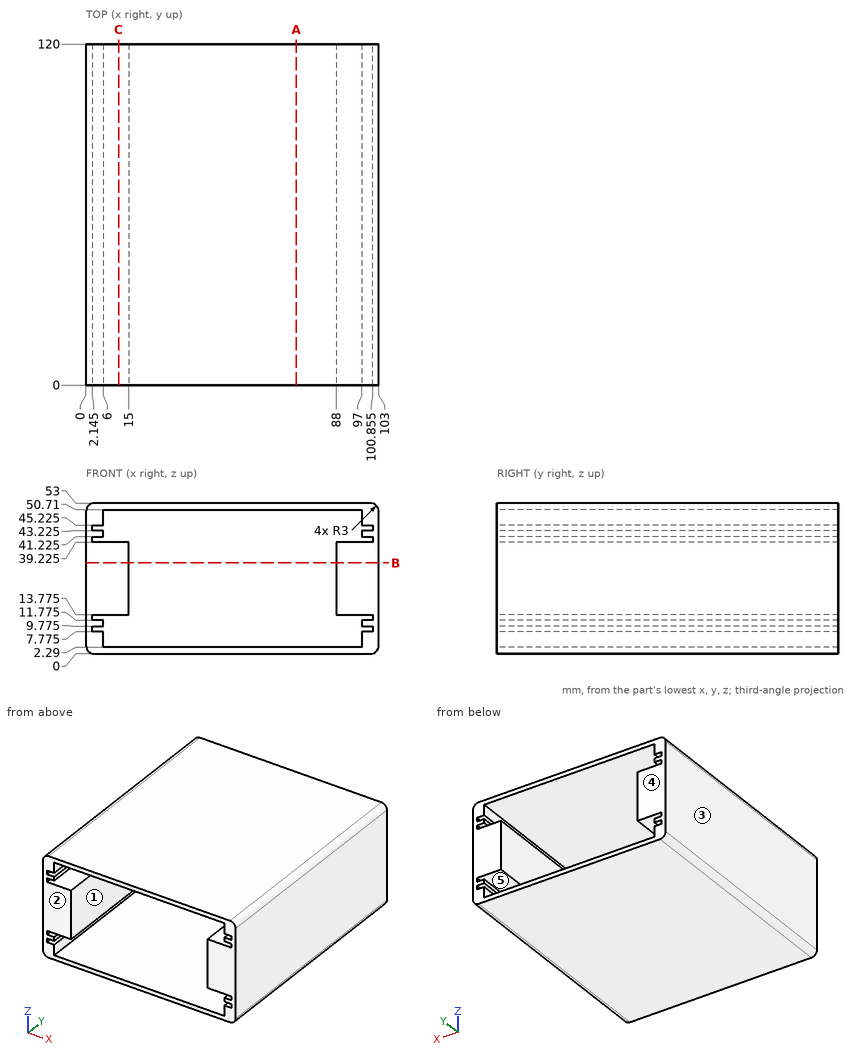
Geometry: see drawing. Coordinates: mm, zero at the bounding-box minimum. A direction names the side the tool comes from. Give positions to 0.01 mm unless a question says otherwise; leave off trailing zeros. Order: outer loops, then holes, each group sorted by start corner. A loop starts at its lowest first (then second) coordinate and runs counter-clockwise, first axis right, second up.
Q1. Draft query along X for the marked faces 1, 2 and 3. Return one class per face: +X half, -X half, draft (parallel to the pull), parting line (faces both ways), or undercut.
Checked values:
face 1: undercut
face 2: draft
face 3: -X half
Q2. Section B-B on z = 32. Output: boundary loops of the cut face in (x, y), and give its area (3 significant figures).
Checked values:
outline: (0, 0) - (15, 0) - (15, 120) - (0, 120) - close; (88, 0) - (103, 0) - (103, 120) - (88, 120) - close
area: 3,600 mm2
Q3. Set-up query: the marked faces 4 and 5. Return all of +Z, -Z, +X, -X, +Y, -Y with unobstructed straight access to the full face (end or side cutting, diameter ignored); none if empty.
Checked values:
face 4: +Z, -Z, +X, -X, +Y
face 5: +Y, -Y
Q4. Ray query, probe 1 along Z at (x, y) = (11, 114) (3 decimals); probe 2 along Z at (x, y) = (5, 32) (3 decimals); probe 3 along Z at (x, y) = (22.5, 94). Return the intervals inside material, ascending.
Checked values:
probe 1: z = 0 to 2.29, 13.775 to 39.225, 50.71 to 53
probe 2: z = 0 to 7.775, 9.775 to 11.775, 13.775 to 39.225, 41.225 to 43.225, 45.225 to 53
probe 3: z = 0 to 2.29, 50.71 to 53
Q5. Section A-A on x = 74. Output: boundary loops of the cut face in (y, z), and give its area (3 significant figures).
Checked values:
outline: (0, 0) - (120, 0) - (120, 2.29) - (0, 2.29) - close; (0, 50.71) - (120, 50.71) - (120, 53) - (0, 53) - close
area: 550 mm2
Q6. Section C-C on x = 11.5. Output: boundary loops of the cut face in (y, z) (3 decimals).
Checked values:
outline: (0, 0) - (120, 0) - (120, 2.29) - (0, 2.29) - close; (0, 13.775) - (120, 13.775) - (120, 39.225) - (0, 39.225) - close; (0, 50.71) - (120, 50.71) - (120, 53) - (0, 53) - close
